The model under review builds one solid part; all positions refer to its coordinate system, in mm. Face numbers are marked on the shaded views. A direction names the side the tool comes from. Give positions to 0.01 mm unless a question says otherwise; leave off trailing zeros. Loops run counter-clockwise (first coordinate to the right, second up) from the corner with the lowest first, then second, coordinate; pieces in that order, holes last. Notation, with made-up numbers: M -9.75,89 L 12.25,89 A14 ccw 12.25,106 Z; hole C 24,13 d4. An arc over 180 degrees is marked long. One line per item, written item: value. Start each with the question number.
Q1. We need section D-D on x = -16.75. Write out the cut boundary in (y, z), plus the area to 3 significant figures.
Q2. To check wall thickness, follow line 1 along Y through (x, z) = (0, -8.05); line 2 along X through (y, z) = (1.5, -5.5). State the ranges of each line that lie inside material, in increasing order. Write a range as from..to.
Q3. Mouldability with a two-part tool opening along Y and no side actions: class the marked faces 1, 2, 3 and 4 as released by +Y, released by -Y, zero draft, split by the parting line, or undercut.
Q4. For the marked faces 5 and 6, list the 3-axis set-ups (+Z, -Z, +X, -X, +Y, -Y) from which the entire face can be reached by the end or side of a thin tool; tool diameter is ignored.
Q5. We need section A-A on y = 0. Write out the cut boundary in (x, z), plus the area to 3 significant figures.
Q6. We need section B-B on x = 0. Write out the cut boundary in (y, z), plus the area to 3 significant figures.
Q7. We need section C-C on z = -2. Write out the cut boundary in (x, y) (3 decimals).
Q8. For pin 1 (12 mm diameter, centred on x = 0, y = 0, fed in from -Z); pin 2 (2 mm diameter, centred on y = 10, z = -1.5, fed in from -X); pin 3 (1 mm diameter, centred on x = 8, y = -14, fed in from +Z); pin 4 (2 mm diameter, centred on y = -4.5, z = -4, fed in from -X), all flat-tipped, find the tip position at first contact; note any pin that passes through.
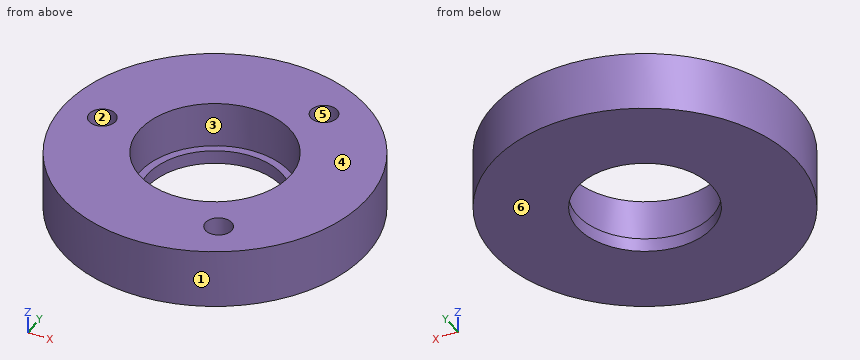
```python
from build123d import *

# Parameters (mm, degrees)
HOLE001_D           = 3.4
HOLE001_DEPTH       = 5
HOLE001_CBORE_D     = 3.9
HOLE001_CBORE_DEPTH = 4
POLARPATTERN_COUNT  = 3


with BuildPart() as part:
    # Sketch003 → Revolution (revolve)
    with BuildSketch(Plane.XZ):
        Polygon((-22.5, 0), (-22.5, -8.75), (-10, -8.75), (-10, -6.75), (-11.15, -6.75), (-11.15, 0), align=None)
    revolve(axis=Axis((0, 0, 0), (0, 0, 1)))

    # Hole001
    with Locations(Plane.XY):
        with Locations((-16.75, 0)):
            hole001 = CounterBoreHole(HOLE001_D / 2, HOLE001_CBORE_D / 2, HOLE001_CBORE_DEPTH, depth=HOLE001_DEPTH)

    # PolarPattern: Hole001 ×3 about axis
    polarpattern_axis = Axis((0, 0, 0), (0, 0, 1))
    for i in range(1, POLARPATTERN_COUNT):
        add(hole001.rotate(polarpattern_axis, i * 360 / POLARPATTERN_COUNT), mode=Mode.SUBTRACT)


solid = part.part
```
Solved:
1. outline: M -15.02,-8.75 L 15.02,-8.75 L 15.02,0 L 1.95,0 L 1.95,-4 L 1.7,-4 L 1.7,-5 L -1.7,-5 L -1.7,-4 L -1.95,-4 L -1.95,0 L -15.02,0 Z
1. area: 244 mm2
2. line 1: -22.5..-10, 10..22.5
2. line 2: -22.45..-11.05, 11.05..22.45
3. face 1: split by the parting line
3. face 2: undercut
3. face 3: undercut
3. face 4: zero draft
4. face 5: +Z
4. face 6: -Z, +X, -X, +Y, -Y
5. outline: M -22.5,-8.75 L -10,-8.75 L -10,-6.75 L -11.15,-6.75 L -11.15,0 L -14.8,0 L -14.8,-4 L -15.05,-4 L -15.05,-5 L -18.45,-5 L -18.45,-4 L -18.7,-4 L -18.7,0 L -22.5,0 Z; M 10,-8.75 L 22.5,-8.75 L 22.5,0 L 11.15,0 L 11.15,-6.75 L 10,-6.75 Z
5. area: 184 mm2
6. outline: M -22.5,-8.75 L -10,-8.75 L -10,-6.75 L -11.15,-6.75 L -11.15,0 L -22.5,0 Z; M 10,-8.75 L 22.5,-8.75 L 22.5,0 L 11.15,0 L 11.15,-6.75 L 10,-6.75 Z
6. area: 203 mm2
7. outline: C 0,0 d45; hole C -16.75,0 d3.9; hole C 0,0 d22.3; hole C 8.375,-14.506 d3.9; hole C 8.375,14.506 d3.9
8. pin 1: through
8. pin 2: x = -20.62
8. pin 3: z = -5
8. pin 4: x = -22.23
